Work out the finished part from the listing and answer in its coordinate system (mm). A direction names the side the tool comes from. Give positions to 0.01 mm unless a question says otherwise; leave off trailing zeros. Loops run counter-clockwise (first coordinate to the right, second up) from the corner with the lowest first, then second, coordinate; pieces in that order, holes last. Notation, with made-up numbers: (-33, -36) - (15, -36) arc R13 ccw to (15, -19) - close; hole circle Ø4 at (-10.5, -4.75). An arc over 180 degrees is marked (long way). One line per item, written item: value.
from build123d import *

# Parameters (mm, degrees)
F0_W     = 3
F0_H     = 10
F1_DEPTH = 15
F0_W_2   = 12
F0_R     = 1.75
F0_W_3   = 7
F2_DEPTH = 3
F3_R     = 2.05
F4_DEPTH = 3
F6_DEPTH = 25.001
F7_R     = 2
F8_R     = 0.5


with BuildPart() as f1:
    # F0 (on Top) → F1 (new body)
    with BuildSketch(Plane.XY):
        Polygon((-43.3751196787, 21.2396075964), (-68.3751196787, 21.2396075964), (-68.3751196787, 18.2396075964), (-65.3751196787, 18.2396075964), (-58.3751196787, 18.2396075964), (-55.3751196787, 18.2396075964), (-43.3751196787, 18.2396075964), align=None)
        with Locations((-66.8751196787, 13.2396075964)):
            Rectangle(F0_W, F0_H)
        with Locations((-56.8751196787, 13.2396075964)):
            Rectangle(F0_W, F0_H)
    extrude(amount=F1_DEPTH)

    # F0 (on Top) → F2 (join)
    with BuildSketch(Plane.XY):
        Polygon((-43.3751196787, 21.2396075964), (-68.3751196787, 21.2396075964), (-68.3751196787, 18.2396075964), (-65.3751196787, 18.2396075964), (-58.3751196787, 18.2396075964), (-55.3751196787, 18.2396075964), (-43.3751196787, 18.2396075964), align=None)
        with Locations((-66.8751196787, 13.2396075964)):
            Rectangle(F0_W, F0_H)
        with Locations((-49.3751196787, 13.2396075964)):
            Rectangle(F0_W_2, F0_H)
        with Locations((-49.3751196787, 12.3196075964)):
            Circle(F0_R, mode=Mode.SUBTRACT)
        with Locations((-61.8751196787, 13.2396075964)):
            Rectangle(F0_W_3, F0_H)
        with Locations((-61.8751196787, 14.5696075964)):
            Circle(F0_R, mode=Mode.SUBTRACT)
        with Locations((-56.8751196787, 13.2396075964)):
            Rectangle(F0_W, F0_H)
    extrude(amount=F2_DEPTH)

    # F3 (on face) → F4 (cut)
    with BuildSketch(Plane.XZ.offset(-18.2396075964)):
        with BuildLine():
            ThreePointArc((-48.3751196787, 15), (-44.8395857727, 13.5355339059), (-43.3751196787, 10))
            Line((-43.3751196787, 10), (-43.3751196787, 15))
            Line((-43.3751196787, 15), (-48.3751196787, 15))
        make_face()
        with Locations((-48.3751196787, 10)):
            Circle(F3_R)
    extrude(amount=-F4_DEPTH, mode=Mode.SUBTRACT)

    # F5 (on face) → F6 (cut, through all)
    with BuildSketch(Plane(origin=(-68.3751196787, 0, 0), x_dir=(0, -1, 0), z_dir=(-1, 0, 0))):
        Polygon((-8.2396075964, 15), (-18.2396075964, 15), (-8.2396075964, 3), align=None)
    extrude(amount=-F6_DEPTH, mode=Mode.SUBTRACT)

    # F7
    f7_edges = [f1.edges().sort_by_distance(p)[0] for p in [
        (-68.37512, 8.239608, 1.5),
        (-43.37512, 8.239608, 1.5),
        (-68.37512, 21.239608, 7.5),
    ]]
    fillet(f7_edges, radius=F7_R)

    # F8
    f8_edges = [f1.edges().sort_by_distance(p)[0] for p in [
        (-55.37512, 13.239608, 3),
        (-49.37512, 18.239608, 3),
        (-55.37512, 18.239608, 9),
        (-65.37512, 13.239608, 3),
        (-61.87512, 18.239608, 3),
        (-65.37512, 18.239608, 9),
        (-58.37512, 18.239608, 9),
        (-58.37512, 13.239608, 3),
    ]]
    fillet(f8_edges, radius=F8_R)


solid = f1.part
1. Section B-B (x = -55.75) is taken. Write down the section's boundary in (y, z).
Output:
outline: (8.24, 0) - (21.24, 0) - (21.24, 15) - (18.24, 15) - (8.24, 3) - close
2. For faces 4 (the flat face through (-65.375, 15, 6)), 5 (the flat face through (-50.5, 14.1, 3)), 6 (the cylindrical face through (-47.76, 11.65, 1.48)), determine the directions among +Z, -Z, +X, -X, +Y, -Y from which every point of the face is accessible in a straight line to the end or side of a thin tool.
Output:
face 4: +Z, -Y
face 5: +Z, +X, -Y
face 6: +Z, -Z
3. Section A-A (z = 9.25) is taken. Write down the section's boundary in (x, y).
Output:
outline: (-68.38, 13.45) - (-65.38, 13.45) - (-65.38, 17.74) arc R0.5 cw to (-64.88, 18.24) - (-58.88, 18.24) arc R0.5 cw to (-58.38, 17.74) - (-58.38, 13.45) - (-55.38, 13.45) - (-55.38, 17.74) arc R0.5 cw to (-54.88, 18.24) - (-50.28, 18.24) - (-50.28, 21.24) - (-66.38, 21.24) arc R2 ccw to (-68.38, 19.24) - close; (-46.47, 18.24) - (-43.38, 18.24) - (-43.38, 21.24) - (-46.47, 21.24) - close
4. Flat-ended cylindrical pins translate along their axes: pin 1 Ø4 at (y, z) = (15, 8) entering from +X; pin 2 Ø6 at (x, z) = (-49, 11.5) entering from -Y; pin 3 Ø3 at (x, y) = (-61.88, 14.57) entering from +Z; pin 4 Ø5 at (x, y) = (-62, 14.5) entering from +Z. Find the tip coordinate at first contact, or state that the pin passes through.
Output:
pin 1: stops at x = -55.38
pin 2: stops at y = 18.24
pin 3: passes through
pin 4: stops at z = 3
5. Find the intervals of material crossed by line 1 along X through (y, z) = (16, 5); line 2 along Y through (x, z) = (-51, 6.25); line 3 along Z through (x, y) = (-64.25, 12.5), in increasing order.
Output:
line 1: x = -68.38 to -65.38, -58.38 to -55.38
line 2: y = 18.24 to 21.24
line 3: z = 0 to 3
6. Section C-C (z = 10.75) is taken. Write down the section's boundary in (x, y), and give its area (3 significant figures).
Output:
outline: (-68.38, 14.7) - (-65.38, 14.7) - (-65.38, 17.74) arc R0.5 cw to (-64.88, 18.24) - (-58.88, 18.24) arc R0.5 cw to (-58.38, 17.74) - (-58.38, 14.7) - (-55.38, 14.7) - (-55.38, 17.74) arc R0.5 cw to (-54.88, 18.24) - (-50.28, 18.24) - (-50.28, 21.24) - (-66.38, 21.24) arc R2 ccw to (-68.38, 19.24) - close; (-46.47, 18.24) - (-43.43, 18.24) - (-43.43, 21.24) - (-46.47, 21.24) - close
area: 83.9 mm²
7. The mould has two halves that part along X. Classify faces 1 (the cylindrical face through (-44.879, 19.719, 13.574)), 2 (the cylindrical face through (-46.481, 19.719, 9.215)), 3 (the flat face through (-55, 21.24, 7)): released by +X, released by -X, zero draft, split by the parting line, or undercut.
Output:
face 1: released by +X
face 2: undercut
face 3: zero draft
8. Section D-D (y = 17) is taken. Write down the section's boundary in (x, z).
Output:
outline: (-68.38, 0) - (-43.38, 0) - (-43.38, 3) - (-54.88, 3) arc R0.5 cw to (-55.38, 3.5) - (-55.38, 13.51) - (-58.38, 13.51) - (-58.38, 3.5) arc R0.5 cw to (-58.88, 3) - (-64.88, 3) arc R0.5 cw to (-65.38, 3.5) - (-65.38, 13.51) - (-68.38, 13.51) - close
